```python
from build123d import *

# Parameters (mm, degrees)
BASE_FLANGE1_START = -184.15
BASE_FLANGE1_DEPTH = 368.3
SKETCH3_R          = 2.1082
CUT_EXTRUDE1_DEPTH = 187.620719687
CUT_EXTRUDE2_DEPTH = 1.016


# Read off the part's stored shape, not the designer's step: Base-Flange1
with BuildPart() as part:
    # Base-Flange1 outline → Base-Flange1 (new body)
    with BuildSketch(Plane(origin=(0, 0, 0), x_dir=(0, 0, -1), z_dir=(1, 0, 0)).offset(BASE_FLANGE1_START)):
        with BuildLine():
            ThreePointArc((-13.368341316, -20.466361674), (-13.309368584, -21.067196652), (-12.979624415, -21.57291321))
            Line((-12.979624415, -21.57291321), (-7.03115395, -27.148026465))
            Line((-7.03115395, -27.148026465), (-6.336374421, -26.406718563))
            Line((-6.336374421, -26.406718563), (-12.284844886, -20.831605308))
            ThreePointArc((-12.284844886, -20.831605308), (-12.350793719, -20.730461996), (-12.362588266, -20.610295001))
            Line((-12.362588266, -20.610295001), (-9.589648917, -1.234016668))
            ThreePointArc((-9.589648917, -1.234016668), (-9.504608121, -1.078094077), (-9.338210654, -1.016))
            Line((-9.338210654, -1.016), (5.562599869, -1.016))
            Line((5.562599869, -1.016), (5.562599869, 0))
            Line((5.562599869, 0), (-9.338210654, 0))
            ThreePointArc((-9.338210654, 0), (-10.170197987, -0.310470387), (-10.595401966, -1.090083341))
            Line((-10.595401966, -1.090083341), (-13.368341316, -20.466361674))
        make_face()
    extrude(amount=BASE_FLANGE1_DEPTH)

    # Sketch3 → Cut-Extrude1 (cut, through all)
    with BuildSketch(Plane(origin=(0, 0, 0), x_dir=(1, 0, 0), z_dir=(0, 1, 0))):
        with Locations(Location((0, 0, 0), (0, 0, 270))):
            Circle(SKETCH3_R)
        with Locations(Location((76.2, 0, 0), (0, 0, 270))):
            Circle(SKETCH3_R)
        with Locations(Location((165.1, 0, 0), (0, 0, 270))):
            Circle(SKETCH3_R)
        with Locations(Location((-165.1, 0, 0), (0, 0, 270))):
            Circle(SKETCH3_R)
        with Locations(Location((-76.2, 0, 0), (0, 0, 270))):
            Circle(SKETCH3_R)
    extrude(amount=-CUT_EXTRUDE1_DEPTH, mode=Mode.SUBTRACT)

    # Sketch4 → Cut-Extrude2 (cut)
    with BuildSketch(Plane(origin=(0, 0, 0), x_dir=(1, 0, 0), z_dir=(0, 1, 0))):
        Polygon((-170.559937336, 6.452662534), (-235.374711333, -58.362111464), (-235.374711333, 6.452662534), align=None)
        Polygon((235.374711333, 6.452662534), (170.559937336, 6.452662534), (235.374711333, -58.362111464), align=None)
    extrude(amount=-CUT_EXTRUDE2_DEPTH, mode=Mode.SUBTRACT)


solid = part.part
```
Input: part model. Units: mm. Frame: model coordinates. A direction names the side the tool comes from. Give positions to 0.01 mm unless a question says otherwise; leave off trailing zeros. Order: outer loops, then holes, each group sorted by start corner. A loop starts at its lowest first (then second) coordinate and runs counter-clockwise, first axis right, second up. Notation, with made-up numbers: M -19.75,85.5 L 26.25,85.5 A35 cw 26.25,118.5 Z; hole C -9,69.5 d9. An arc over 180 degrees is marked long. Return JSON: item names as keys, results as strings.
Item 1: Cut plane B-B (y = -5). Return loops of the section in (x, z).
Solutions:
{"outline": "M -184.15,10.13 L 184.15,10.13 L 184.15,11.15 L -184.15,11.15 Z"}
Item 2: Access query for faces 1 (the flat face through (-2.58, -24.32, 10.05)), 2 (the flat face through (-3, -1.016, 2)). Directions: +Z, -Z, +X, -X, +Y, -Y. A direction counts if a zero-diameter tool reaches every point of the face in a straight line with its end or side. Return the directions, or none.
Solutions:
{"face 1": "+Z, +X, -X, -Y", "face 2": "-Z, +X, -X"}
Item 3: Cut plane A-A (x = -133.5). Return loops of the section in (y, z).
Solutions:
{"outline": "M -27.15,7.03 L -26.41,6.34 L -20.83,12.28 A0.25 cw -20.61,12.36 L -1.23,9.59 A0.25 cw -1.02,9.34 L -1.02,-5.56 L 0,-5.56 L 0,9.34 A1.27 ccw -1.09,10.6 L -20.47,13.37 A1.27 ccw -21.57,12.98 Z"}
Item 4: Pull-direction query (Y, two-part tool) for faces 3 (the flat face through (-3, 0, 2)), 4 (the flat face through (-2.578, -23.658, 9.269)), 5 (the flat face through (184.15, -14, 12)), 6 (the flat face through (-2.6, -11.1, 11)); classes: +Y half, -Y half, draft (parallel to the pull), parting line (faces both ways), or undercut.
Solutions:
{"face 3": "+Y half", "face 4": "undercut", "face 5": "draft", "face 6": "undercut"}
Item 5: First-contact query: P1, Ø10, axis at y = -20, z = 1.5, coming from the -X side; P2, Ø1, axis at x = -4.5, z = 5.5, coming from the -Y side; P3, Ø2, axis at x = 128.5, y = -23.5, coming from the -Z side; P4, Ø2, axis at x = 45, y = -14, coming from the +Z side. Flat tips, straight axial feed; report the tip coordinate or a pass-through.
Solutions:
{"P1": "through", "P2": "y = -1.02", "P3": "z = 8.37", "P4": "z = 12.59"}
Item 6: Ray query, probe 1 along X at (y, z) = (-0.55, 0); probe 2 along Y at (x, z) = (-79.5, 2); probe 3 along Y at (x, z) = (113, 9.25). Return the intervals inside material, ascending.
Solutions:
{"probe 1": "-177.01 to -167.21, -162.99 to -78.31, -74.09 to -2.11, 2.11 to 74.09, 78.31 to 162.99, 167.21 to 177.01", "probe 2": "-1.02 to 0", "probe 3": "-25.07 to -23.68, -1.02 to 0"}
